Verification items for the finished model (mm, model axes). Round coordinates to 2 decimals unless told otherwise and drop trailing zeros. Return JSON: item names as keys, results as strings. Group by question number.
Item 1: Depth check by flat-ended pin: pin 1 Ø5 at (x, y) = (1.5, -17) entering from +Z; pin 2 Ø10 at (x, y) = (-25.5, -4) entering from -Z; pin 3 Ø1 at (y, z) = (-3.5, -25) entering from +X. Enter the tip coordinate at first touch or a pass-through.
Item 2: Scan lines: probe 1 along X at (y, z) = (-7.25, -7); probe 2 along X at (y, z) = (-1.25, -3.5); probe 3 along X at (y, z) = (-22, -26). Record each from-to range of solid material in increasing order. Write a range as from..to.
Item 3: Draft check along X on faces 1 (the flat face through (-1, -25.4, -16)), 2 (the flat face through (-51.16, -12.52, -8.18)), 3 (the cylindrical face through (0.311, -11.768, -13.667)), 4 (the flat face through (51.126, -12.522, -8.415)). Enter one of: pulls with the +X half, pulls with the -X half, needs draft (parallel to the pull), parting line crosses it, or undercut.
```python
from build123d import *

# Parameters (mm, degrees)
F1_DEPTH = 25.4
F3_R     = 12.065
F4_DEPTH = 76.2


with BuildPart() as f1:
    # F0 (on Front) → F1 (new body)
    with BuildSketch(Plane.XZ):
        with BuildLine():
            Line((52.3875, 0), (-52.3875, 0))
            Line((-52.3875, 0), (-49.8988601972, -16.5985570235))
            add(Edge.make_bspline(
                [(-49.8988601972, -16.5985570235), (-49.8988601972, -19.9378890599), (-6.0647983403, -16.1415340845), (-5.8959199742, -32.0347056309), (0, -32.349884783)],
                knots=[0, 0, 0, 0, 0.6030923859, 1, 1, 1, 1], degree=3))
            add(Edge.make_bspline(
                [(49.8988601972, -16.5985570235), (49.8988601972, -19.9378890599), (6.0647983403, -16.1415340845), (5.8959199742, -32.0347056309), (0, -32.349884783)],
                knots=[0, 0, 0, 0, 0.6030923859, 1, 1, 1, 1], degree=3))
            Line((49.8988601972, -16.5985570235), (52.3875, 0))
        make_face()
    extrude(amount=F1_DEPTH)

    # F3 (on face) → F4 (cut)
    with BuildSketch(Plane(origin=(0, 0, 0), x_dir=(-1, 0, 0), z_dir=(0, 0.9918944426, 0.1270646086))):
        Circle(F3_R)
    extrude(amount=-F4_DEPTH, mode=Mode.SUBTRACT)


solid = f1.part
```
Recorded:
{
 "1": {"pin 1": "z = -13.6", "pin 2": "z = -20.41", "pin 3": "x = 9.75"},
 "2": {"probe 1": "-51.34..-10.45, 10.45..51.34", "probe 2": "-51.86..-11.6, 11.6..51.86", "probe 3": "-8.17..8.17"},
 "3": {"face 1": "needs draft", "face 2": "pulls with the -X half", "face 3": "undercut", "face 4": "pulls with the +X half"}
}
